Read the model definition and answer for the solid it produces. Units are mm, in the model's axes. Face numbers are marked on the shaded views. A direction names the side the tool comes from. Round coordinates to 2 decimals unless told otherwise and drop trailing zeros. Order: outer loops, then holes, each group sorted by start corner. A loop starts at its lowest first (then second) coordinate and runs counter-clockwise, first axis right, second up.
from build123d import *

# Parameters (mm, degrees)
SKETCH1_R                  = 8
SKETCH1_R_2                = 4
BOSS_EXTRUDE1_DEPTH        = 5
SKETCH2_R                  = 16
SKETCH2_R_2                = 4
BOSS_EXTRUDE2_DEPTH        = 3
M4X0_7_TAPPED_HOLE1_REACH  = 31.933
M4X0_7_TAPPED_HOLE1_BORE_R = 1.65
M4_CLEARANCE_HOLE1_D       = 4.5


with BuildPart() as part:
    # Sketch1 → Boss-Extrude1 (new, symmetric)
    with BuildSketch(Plane(origin=(0, 0, 0), x_dir=(1, 0, 0), z_dir=(0, 1, 0))):
        with Locations(Location((0, 0, 0), (0, 0, 270))):
            Circle(SKETCH1_R)
        with Locations(Location((0, 0, 0), (0, 0, 270))):
            Circle(SKETCH1_R_2, mode=Mode.SUBTRACT)
    extrude(amount=BOSS_EXTRUDE1_DEPTH, both=True)

    # Sketch2 → Boss-Extrude2 (add)
    with BuildSketch(Plane(origin=(0, 5, 0), x_dir=(1, 0, 0), z_dir=(0, 1, 0))):
        with Locations(Location((0, 0, 0), (0, 0, 270))):
            Circle(SKETCH2_R)
        with Locations(Location((0, 0, 0), (0, 0, 270))):
            Circle(SKETCH2_R_2, mode=Mode.SUBTRACT)
    extrude(amount=BOSS_EXTRUDE2_DEPTH)

    # M4x0.7 Tapped Hole1 bore → M4x0.7 Tapped Hole1 (cut, up to next)
    with BuildSketch(Plane.ZY.offset(8), mode=Mode.PRIVATE) as m4x0_7_tapped_hole1_sk1:
        Circle(M4X0_7_TAPPED_HOLE1_BORE_R)
    m4x0_7_tapped_hole1_tool1 = extrude(m4x0_7_tapped_hole1_sk1.sketch, amount=-M4X0_7_TAPPED_HOLE1_REACH, mode=Mode.PRIVATE) & part.part
    add(m4x0_7_tapped_hole1_tool1.solids().sort_by_distance((-8, 0, 0))[0], mode=Mode.SUBTRACT)

    # M4 Clearance Hole1 (through all)
    with Locations(Plane(origin=(0, 8, 0), x_dir=(1, 0, 0), z_dir=(0, 1, 0))):
        with Locations((0, 12), (12, 0), (-12, 0), (0, -12)):
            Hole(M4_CLEARANCE_HOLE1_D / 2)


solid = part.part
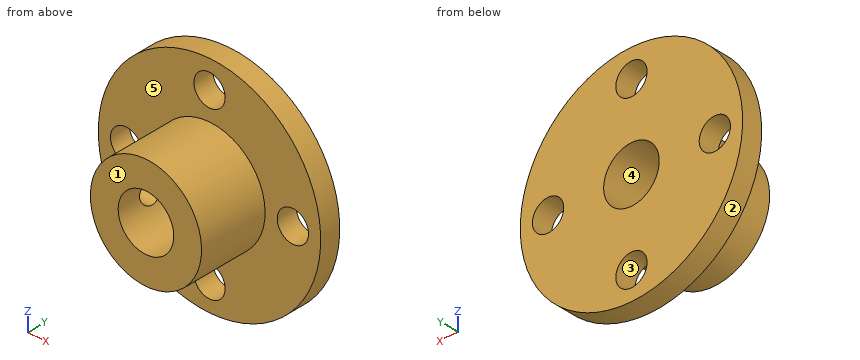
Q1. A cutting plane is placed at A-A, the plane z = 0. Give the vertices of the cut face in (x, y).
Outcome:
outline: (-16, 5) - (-14.25, 5) - (-14.25, 8) - (-16, 8) - close; (-9.75, 5) - (-8, 5) - (-8, 1.65) - (-4, 1.65) - (-4, 8) - (-9.75, 8) - close; (-8, -5) - (-4, -5) - (-4, -1.65) - (-8, -1.65) - close; (4, -5) - (8, -5) - (8, 5) - (9.75, 5) - (9.75, 8) - (4, 8) - close; (14.25, 5) - (16, 5) - (16, 8) - (14.25, 8) - close
Q2. For the marked faces 4 and 5, determine the directions among +Z, -Z, +X, -X, +Y, -Y from which every point of the face is accessible in a straight line to the end or side of a thin tool.
Outcome:
face 4: +Y, -Y
face 5: -Y
Q3. A cutting plane is placed at B-B, the plane x = 0. Give the vertices of the cut face in (y, z), plus the area to 3 significant figures.
Outcome:
outline: (-5, -8) - (5, -8) - (5, -9.75) - (8, -9.75) - (8, -4) - (-5, -4) - close; (-5, 4) - (8, 4) - (8, 9.75) - (5, 9.75) - (5, 8) - (-5, 8) - close; (5, -16) - (8, -16) - (8, -14.25) - (5, -14.25) - close; (5, 14.25) - (8, 14.25) - (8, 16) - (5, 16) - close
area: 125 mm2
Q4. Straight lines are drawn through the part: probe 1 along Y at (x, z) = (-4.55, 0); probe 2 along X at (y, z) = (6.6, 12); probe 3 along Z at (x, y) = (-2, -3). For each, find the intervals that lie inside material, in ascending order.
Outcome:
probe 1: y = -5 to -1.65, 1.65 to 8
probe 2: x = -10.58 to -2.25, 2.25 to 10.58
probe 3: z = -7.75 to -3.46, 3.46 to 7.75
Q5. Flat-ended cylindrical pins translate along their axes: pin 1 (8 mm diameter, centred on x = -11, z = 12.5, fed in from -Y); pin 2 (1 mm diameter, centred on x = -6.5, y = -0.5, fed in from +Z); pin 3 (5 mm diameter, centred on y = 3, z = -5.5, fed in from -X). Find the tip coordinate at first contact, or state that the pin passes through.
Outcome:
pin 1: stops at y = 5
pin 2: stops at z = 5.29
pin 3: stops at x = -15.49
Q6. A cutting plane is placed at C-C, the plane x = 10.5. Give the vertices of the cut face in (y, z), plus the area to 3 significant figures.
Outcome:
outline: (5, -12.07) - (8, -12.07) - (8, -1.68) - (5, -1.68) - close; (5, 1.68) - (8, 1.68) - (8, 12.07) - (5, 12.07) - close
area: 62.4 mm2
Q7. A cutting plane is placed at D-D, the plane z = -11. Give the vertices of the cut face in (x, y), plus the area to 3 significant figures.
Outcome:
outline: (-11.62, 5) - (-2.02, 5) - (-2.02, 8) - (-11.62, 8) - close; (2.02, 5) - (11.62, 5) - (11.62, 8) - (2.02, 8) - close
area: 57.6 mm2
Q8. For a pull along X with two mould halves and no side action, classify the marked faces 1, 2 and 3 as released by +X, released by -X, zero draft, split by the parting line, or undercut.
Outcome:
face 1: zero draft
face 2: split by the parting line
face 3: undercut
